Input: part model. Units: mm. Frame: model coordinates. Face numbers are marked on the shaded views. Coordinates: 2 decimals unless noted, no trailing zeros. Order: outer loops, then holes, each group sorted by start corner. A loop starts at its lowest first (then second) coordinate and runs counter-clockwise, first axis right, second up. Notation, with made-up numbers: (44.25, 21.25) -> (71.25, 21.25) arc R14 ccw to (71.25, 31.25) -> close; hole circle Ø11 at (23.5, 60.25). An arc over 180 degrees is marked (long way). Answer as CSV lines item,"result".
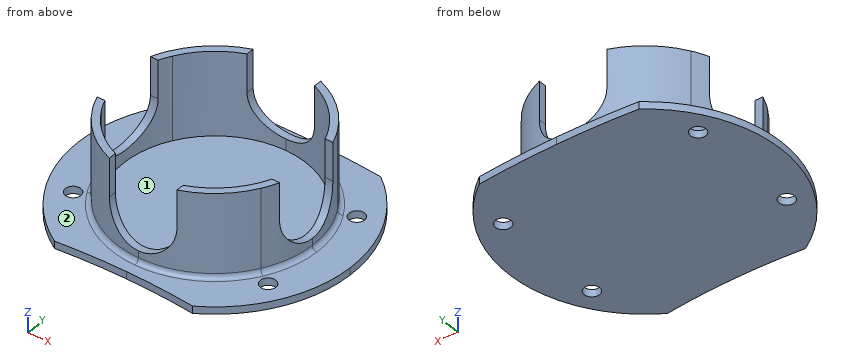
from build123d import *

# Parameters (mm, degrees)
F1_DEPTH  = 2.032
F2_DEPTH  = 25.4
F3_D      = 4.318
F3_DEPTH  = 5.08
F3_TIP    = 1.2972580765
F6_DEPTH  = 63.5
F10_DEPTH = 63.5
F11_R     = 1.27


with BuildPart() as f1:
    # F0 (on Top) → F1 (new body)
    with BuildSketch(Plane.XY):
        with BuildLine():
            ThreePointArc((-19.4727464049, 189.5021428571), (-9.7491483145, 190.2503721603), (0, 190.5))
            ThreePointArc((0, 190.5), (-15.875, 194.7536934298), (-27.4963065702, 206.375))
            ThreePointArc((-27.4963065702, 206.375), (-31.75, 222.25), (-27.4963065702, 238.125))
            ThreePointArc((-27.4963065702, 238.125), (-15.875, 249.7463065702), (0, 254))
            ThreePointArc((0, 254), (-11.2573468074, 253.750413089), (-22.4925700998, 253.0021428571))
            ThreePointArc((-22.4925700998, 253.0021428571), (-38.0569894676, 220.440151204), (-19.4727464049, 189.5021428571))
        make_face()
        with BuildLine():
            Line((0, 249.682), (0, 254))
            ThreePointArc((0, 254), (-15.875, 249.7463065702), (-27.4963065702, 238.125))
            Line((-27.4963065702, 238.125), (-23.7568088766, 235.966))
            ThreePointArc((-23.7568088766, 235.966), (-13.716, 246.0068088766), (0, 249.682))
        make_face()
        with BuildLine():
            ThreePointArc((-27.4963065702, 238.125), (-31.75, 222.25), (-27.4963065702, 206.375))
            Line((-27.4963065702, 206.375), (-23.7568088766, 208.534))
            ThreePointArc((-23.7568088766, 208.534), (-27.432, 222.25), (-23.7568088766, 235.966))
            Line((-23.7568088766, 235.966), (-27.4963065702, 238.125))
        make_face()
        with BuildLine():
            ThreePointArc((-23.7568088766, 235.966), (-27.432, 222.25), (-23.7568088766, 208.534))
            Line((-23.7568088766, 208.534), (-21.9970452561, 209.55))
            ThreePointArc((-21.9970452561, 209.55), (-25.4, 222.25), (-21.9970452561, 234.95))
            Line((-21.9970452561, 234.95), (-23.7568088766, 235.966))
        make_face()
        with BuildLine():
            ThreePointArc((-27.4963065702, 206.375), (-15.875, 194.7536934298), (0, 190.5))
            Line((0, 190.5), (0, 194.818))
            ThreePointArc((0, 194.818), (-13.716, 198.4931911234), (-23.7568088766, 208.534))
            Line((-23.7568088766, 208.534), (-27.4963065702, 206.375))
        make_face()
        with BuildLine():
            ThreePointArc((-23.7568088766, 208.534), (-13.716, 198.4931911234), (0, 194.818))
            Line((0, 194.818), (0, 196.85))
            ThreePointArc((0, 196.85), (-12.7, 200.2529547439), (-21.9970452561, 209.55))
            Line((-21.9970452561, 209.55), (-23.7568088766, 208.534))
        make_face()
        with BuildLine():
            ThreePointArc((-21.9970452561, 209.55), (-12.7, 200.2529547439), (0, 196.85))
            Line((0, 196.85), (0, 222.25))
            Line((0, 222.25), (-21.9970452561, 209.55))
        make_face()
        with BuildLine():
            Line((-21.9970452561, 209.55), (0, 222.25))
            Line((0, 222.25), (-21.9970452561, 234.95))
            ThreePointArc((-21.9970452561, 234.95), (-25.4, 222.25), (-21.9970452561, 209.55))
        make_face()
        with BuildLine():
            Line((-21.9970452561, 234.95), (0, 222.25))
            Line((0, 222.25), (0, 247.65))
            ThreePointArc((0, 247.65), (-12.7, 244.2470452561), (-21.9970452561, 234.95))
        make_face()
        with BuildLine():
            Line((0, 247.65), (0, 249.682))
            ThreePointArc((0, 249.682), (-13.716, 246.0068088766), (-23.7568088766, 235.966))
            Line((-23.7568088766, 235.966), (-21.9970452561, 234.95))
            ThreePointArc((-21.9970452561, 234.95), (-12.7, 244.2470452561), (0, 247.65))
        make_face()
        with BuildLine():
            ThreePointArc((27.4963065702, 238.125), (15.875, 249.7463065702), (0, 254))
            Line((0, 254), (0, 249.682))
            ThreePointArc((0, 249.682), (13.716, 246.0068088766), (23.7568088766, 235.966))
            Line((23.7568088766, 235.966), (27.4963065702, 238.125))
        make_face()
        with BuildLine():
            ThreePointArc((23.7568088766, 235.966), (13.716, 246.0068088766), (0, 249.682))
            Line((0, 249.682), (0, 247.65))
            ThreePointArc((0, 247.65), (12.7, 244.2470452561), (21.9970452561, 234.95))
            Line((21.9970452561, 234.95), (23.7568088766, 235.966))
        make_face()
        with BuildLine():
            Line((0, 247.65), (0, 222.25))
            Line((0, 222.25), (21.9970452561, 234.95))
            ThreePointArc((21.9970452561, 234.95), (12.7, 244.2470452561), (0, 247.65))
        make_face()
        with BuildLine():
            ThreePointArc((0, 190.5), (9.7491483145, 190.2503721603), (19.4727464049, 189.5021428571))
            ThreePointArc((19.4727464049, 189.5021428571), (33.1173794104, 203.4125590648), (38.1, 222.25))
            ThreePointArc((38.1, 222.25), (33.9748209767, 239.493014226), (22.4925700998, 253.0021428571))
            ThreePointArc((22.4925700998, 253.0021428571), (11.2573468074, 253.750413089), (0, 254))
            ThreePointArc((0, 254), (15.875, 249.7463065702), (27.4963065702, 238.125))
            ThreePointArc((27.4963065702, 238.125), (30.6681449847, 230.467504682), (31.75, 222.25))
            ThreePointArc((31.75, 222.25), (30.6681449847, 214.032495318), (27.4963065702, 206.375))
            ThreePointArc((27.4963065702, 206.375), (15.875, 194.7536934298), (0, 190.5))
        make_face()
        with BuildLine():
            Line((23.7568088766, 208.534), (27.4963065702, 206.375))
            ThreePointArc((27.4963065702, 206.375), (30.6681449847, 214.032495318), (31.75, 222.25))
            ThreePointArc((31.75, 222.25), (30.6681449847, 230.467504682), (27.4963065702, 238.125))
            Line((27.4963065702, 238.125), (23.7568088766, 235.966))
            ThreePointArc((23.7568088766, 235.966), (26.4972772668, 229.3499240453), (27.432, 222.25))
            ThreePointArc((27.432, 222.25), (26.4972772668, 215.1500759547), (23.7568088766, 208.534))
        make_face()
        with BuildLine():
            Line((21.9970452561, 209.55), (23.7568088766, 208.534))
            ThreePointArc((23.7568088766, 208.534), (26.4972772668, 215.1500759547), (27.432, 222.25))
            ThreePointArc((27.432, 222.25), (26.4972772668, 229.3499240453), (23.7568088766, 235.966))
            Line((23.7568088766, 235.966), (21.9970452561, 234.95))
            ThreePointArc((21.9970452561, 234.95), (24.5345159877, 228.8240037456), (25.4, 222.25))
            ThreePointArc((25.4, 222.25), (24.5345159877, 215.6759962544), (21.9970452561, 209.55))
        make_face()
        with BuildLine():
            Line((21.9970452561, 234.95), (0, 222.25))
            Line((0, 222.25), (21.9970452561, 209.55))
            ThreePointArc((21.9970452561, 209.55), (24.5345159877, 215.6759962544), (25.4, 222.25))
            ThreePointArc((25.4, 222.25), (24.5345159877, 228.8240037456), (21.9970452561, 234.95))
        make_face()
        with BuildLine():
            Line((0, 222.25), (0, 196.85))
            ThreePointArc((0, 196.85), (12.7, 200.2529547439), (21.9970452561, 209.55))
            Line((21.9970452561, 209.55), (0, 222.25))
        make_face()
        with BuildLine():
            Line((0, 196.85), (0, 194.818))
            ThreePointArc((0, 194.818), (13.716, 198.4931911234), (23.7568088766, 208.534))
            Line((23.7568088766, 208.534), (21.9970452561, 209.55))
            ThreePointArc((21.9970452561, 209.55), (12.7, 200.2529547439), (0, 196.85))
        make_face()
        with BuildLine():
            Line((0, 194.818), (0, 190.5))
            ThreePointArc((0, 190.5), (15.875, 194.7536934298), (27.4963065702, 206.375))
            Line((27.4963065702, 206.375), (23.7568088766, 208.534))
            ThreePointArc((23.7568088766, 208.534), (13.716, 198.4931911234), (0, 194.818))
        make_face()
    extrude(amount=F1_DEPTH)

    # F0 (on Top) → F2 (join)
    with BuildSketch(Plane.XY):
        with BuildLine():
            ThreePointArc((-23.7568088766, 208.534), (-13.716, 198.4931911234), (0, 194.818))
            Line((0, 194.818), (0, 196.85))
            ThreePointArc((0, 196.85), (-12.7, 200.2529547439), (-21.9970452561, 209.55))
            Line((-21.9970452561, 209.55), (-23.7568088766, 208.534))
        make_face()
        with BuildLine():
            ThreePointArc((-23.7568088766, 235.966), (-27.432, 222.25), (-23.7568088766, 208.534))
            Line((-23.7568088766, 208.534), (-21.9970452561, 209.55))
            ThreePointArc((-21.9970452561, 209.55), (-25.4, 222.25), (-21.9970452561, 234.95))
            Line((-21.9970452561, 234.95), (-23.7568088766, 235.966))
        make_face()
        with BuildLine():
            Line((0, 247.65), (0, 249.682))
            ThreePointArc((0, 249.682), (-13.716, 246.0068088766), (-23.7568088766, 235.966))
            Line((-23.7568088766, 235.966), (-21.9970452561, 234.95))
            ThreePointArc((-21.9970452561, 234.95), (-12.7, 244.2470452561), (0, 247.65))
        make_face()
        with BuildLine():
            ThreePointArc((23.7568088766, 235.966), (13.716, 246.0068088766), (0, 249.682))
            Line((0, 249.682), (0, 247.65))
            ThreePointArc((0, 247.65), (12.7, 244.2470452561), (21.9970452561, 234.95))
            Line((21.9970452561, 234.95), (23.7568088766, 235.966))
        make_face()
        with BuildLine():
            Line((21.9970452561, 209.55), (23.7568088766, 208.534))
            ThreePointArc((23.7568088766, 208.534), (26.4972772668, 215.1500759547), (27.432, 222.25))
            ThreePointArc((27.432, 222.25), (26.4972772668, 229.3499240453), (23.7568088766, 235.966))
            Line((23.7568088766, 235.966), (21.9970452561, 234.95))
            ThreePointArc((21.9970452561, 234.95), (24.5345159877, 228.8240037456), (25.4, 222.25))
            ThreePointArc((25.4, 222.25), (24.5345159877, 215.6759962544), (21.9970452561, 209.55))
        make_face()
        with BuildLine():
            Line((0, 196.85), (0, 194.818))
            ThreePointArc((0, 194.818), (13.716, 198.4931911234), (23.7568088766, 208.534))
            Line((23.7568088766, 208.534), (21.9970452561, 209.55))
            ThreePointArc((21.9970452561, 209.55), (12.7, 200.2529547439), (0, 196.85))
        make_face()
    extrude(amount=F2_DEPTH)

    # F3
    with Locations(Plane(origin=(0, 0, 0), x_dir=(1, 0, 0), z_dir=(0, 0, -1))):
        with Locations((-27.4963065702, -206.375), (-27.4963065702, -238.125), (27.4963065702, -238.125), (27.4963065702, -206.375)):
            Hole(F3_D / 2, depth=F3_DEPTH)
            with Locations((0, 0, -(F3_DEPTH + F3_TIP / 2))):  # 118° drill point
                Cone(0, F3_D / 2, F3_TIP, mode=Mode.SUBTRACT)

    # F5 (on line) → F6 (cut, symmetric)
    with BuildSketch(Plane.YZ):
        with BuildLine():
            Line((212.725, 28.6151301116), (212.725, 14.732))
            ThreePointArc((212.725, 14.732), (215.5148079092, 7.9968079092), (222.25, 5.207))
            ThreePointArc((222.25, 5.207), (228.9851920908, 7.9968079092), (231.775, 14.732))
            Line((231.775, 14.732), (231.775, 28.6151301116))
            Line((231.775, 28.6151301116), (212.725, 28.6151301116))
        make_face()
    extrude(amount=F6_DEPTH, both=True, mode=Mode.SUBTRACT)

    # F9 (on line) → F10 (cut, symmetric)
    with BuildSketch(Plane.XZ.offset(-222.25)):
        with BuildLine():
            Line((-9.525, 30.1762204617), (-9.525, 14.732))
            ThreePointArc((-9.525, 14.732), (-6.7351920908, 7.9968079092), (0, 5.207))
            ThreePointArc((0, 5.207), (6.7351920908, 7.9968079092), (9.525, 14.732))
            Line((9.525, 14.732), (9.525, 30.1762204617))
            Line((9.525, 30.1762204617), (-9.525, 30.1762204617))
        make_face()
    extrude(amount=F10_DEPTH, both=True, mode=Mode.SUBTRACT)

    # F11
    f11_edges = [f1.edges().sort_by_distance(p)[0] for p in [
        (0, 249.682, 2.032),
    ]]
    fillet(f11_edges, radius=F11_R)


solid = f1.part
1. Ray query, line 1 along Z through (x, y) = (24.5, 237); line 2 along Y through (x, z) = (12, 12.25); line 3 along X through (y, z) = (205, 24). Return the intervals inside material, ascending.
Findings:
line 1,"z = 0 to 2.04"
line 2,"y = 197.58 to 199.86, 244.64 to 246.92"
line 3,"x = -21.33 to -18.64, 18.64 to 21.33"
2. Mould query, pull axis X, two halves, no side actions, for the marked faces 1 and 2. Classes: released by +X, released by -X, zero draft, split by the parting line, or undercut.
Findings:
face 1,"undercut"
face 2,"zero draft"
3. Cut plane B-B (z = 7). Return the cut outline in (x, y), plus the area to 3 significant figures.
Findings:
outline,"(-26.86, 216.69) arc R27.43 ccw to (-5.56, 195.39) -> (-5.56, 197.47) arc R25.4 cw to (-24.78, 216.69) -> close; (-26.86, 227.81) -> (-24.78, 227.81) arc R25.4 cw to (-5.56, 247.03) -> (-5.56, 249.11) arc R27.43 ccw to start; (5.56, 195.39) arc R27.43 ccw to (26.86, 216.69) -> (24.78, 216.69) arc R25.4 cw to (5.56, 197.47) -> close; (5.56, 247.03) arc R25.4 cw to (24.78, 227.81) -> (26.86, 227.81) arc R27.43 ccw to (5.56, 249.11) -> close"
area,"246 mm2"
4. Contact query for flat-ended pins moving along their axis: pin 1 (5.5 mm diameter, centred on x = 27.5, y = 238.12, fed in from +Z); pin 2 (1 mm diameter, centred on y = 247, z = 17.5, fed in from -X); pin 3 (1.7 mm diameter, centred on y = 247, z = 19, fed in from +X); pin 4 (4 mm diameter, centred on x = 27.5, y = 206.38, fed in from -Z). Output: stop coordinate, or through.
Findings:
pin 1,"stops at z = 2.03"
pin 2,"stops at x = -12.82"
pin 3,"stops at x = 13.46"
pin 4,"passes through"
5. Cut plane A-A (z = 23.25). Return the cut outline in (x, y) (3 decimals), plus the area to 3 significant figures.
Findings:
outline,"(-25.725, 212.725) arc R27.432 ccw to (-9.525, 196.525) -> (-9.525, 198.704) arc R25.4 cw to (-23.546, 212.725) -> close; (-25.725, 231.775) -> (-23.546, 231.775) arc R25.4 cw to (-9.525, 245.796) -> (-9.525, 247.975) arc R27.432 ccw to start; (9.525, 196.525) arc R27.432 ccw to (25.725, 212.725) -> (23.546, 212.725) arc R25.4 cw to (9.525, 198.704) -> close; (9.525, 245.796) arc R25.4 cw to (23.546, 231.775) -> (25.725, 231.775) arc R27.432 ccw to (9.525, 247.975) -> close"
area,"179 mm2"
6. Cut plane C-C (x = -30.5). Return the cut outline in (y, z), plus the area to 3 significant figures.
Findings:
outline,"(199.42, 0) -> (245.08, 0) -> (245.08, 2.03) -> (199.42, 2.03) -> close"
area,"92.8 mm2"
